Input: dimensioned drawing with shaded views. Units: mm. Origin: part minimum x, y, z. Coordinates: 2 decimals unless noted, no trailing zeros. Write each loop counter-clockwise with the first axis right and the second up, starting at its lowest first coordinate (ties: lowest second). Pieces come first, ordered by that corner, then holes. Notation, with made-up numbers: (-15.5, -29.5) - (4.5, -29.5) arc R15 cw to (4.5, -23.5) - close; hole circle Ø1 at (-11, 13.25). An arc over 180 degrees is marked (long way). One line per question, with ' | ' between items.
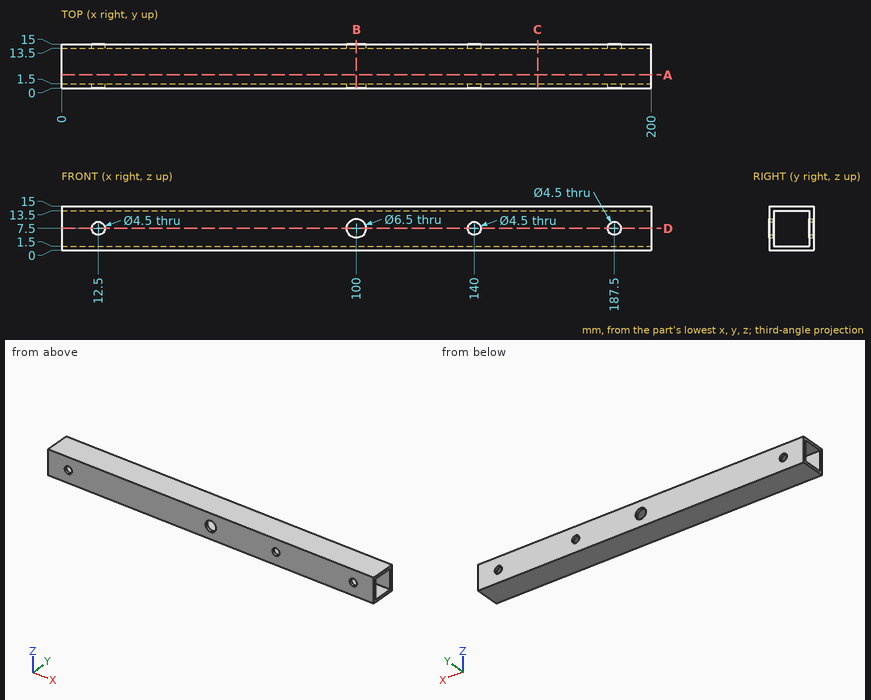
Item 1: Cut plane D-D on z = 7.5. State how many separate pieces and enclosed holes the cut face has, and give its area (3 significant figures).
Check sheet entries:
separate pieces: 10 | enclosed holes: 0 | area: 540 mm²
Item 2: Cut plane A-A on y = 4.5. Return loops of the section in (x, z).
Check sheet entries:
outline: (0, 0) - (200, 0) - (200, 1.5) - (0, 1.5) - close; (0, 13.5) - (200, 13.5) - (200, 15) - (0, 15) - close
Item 3: Cut plane C-C on x = 161.5. Return loops of the section in (y, z), and give its area (3 significant figures).
Check sheet entries:
outline: (0, 0) - (15, 0) - (15, 15) - (0, 15) - close; hole (1.5, 1.5) - (13.5, 1.5) - (13.5, 13.5) - (1.5, 13.5) - close | area: 81.0 mm²
Item 4: Ray query, line 1 along X through (y, z) = (14, 7.5); line 2 along Y through (x, z) = (89.5, 7.25). Return the intervals inside material, ascending. Write a range as [from, to].
Check sheet entries:
line 1: [0, 10.25], [14.75, 96.75], [103.25, 137.75], [142.25, 185.25], [189.75, 200] | line 2: [0, 1.5], [13.5, 15]
Item 5: Cut plane B-B on x = 100. Return loops of the section in (y, z), and give its area (3 significant figures).
Check sheet entries:
outline: (0, 0) - (15, 0) - (15, 4.25) - (13.5, 4.25) - (13.5, 1.5) - (1.5, 1.5) - (1.5, 4.25) - (0, 4.25) - close; (0, 10.75) - (1.5, 10.75) - (1.5, 13.5) - (13.5, 13.5) - (13.5, 10.75) - (15, 10.75) - (15, 15) - (0, 15) - close | area: 61.5 mm²
